from build123d import *

# Parameters (mm, degrees)
BOTTOM_PLATE_W                       = 140
BOTTOM_PLATE_H                       = 110
BOTTOM_PLATE_EXT_DEPTH               = 2
TOP_ROW_R                            = 8.25
TOP_ROW_R_2                          = 6.5
TOP_ROW_CUT_DEPTH                    = 179.056170912
SKETCH2_R                            = 6.5
SKETCH2_R_2                          = 3.55
BOTTOM_ROW_CUT_DEPTH                 = 10
SKETCH3_R                            = 6.5
CENTER_ROW_CUT_DEPTH                 = 10
PLATE_SCREWS_R                       = 1.65
PLATE_SCREWS_CUT_DEPTH               = 179.056170912
PLATE_SCREW_HEAD_R                   = 2.8
PLATE_SCREW_HEAD_CUT_DEPTH           = 2
PLATE_SCREW_HEAD_CUT_DRAFT           = -45
PLATE_SCREW_HEAD_CUT_PROFILE_2_DEPTH = 2
PLATE_SCREW_HEAD_CUT_PROFILE_2_DRAFT = -45
PLATE_SCREW_HEAD_CUT_PROFILE_3_DEPTH = 2
PLATE_SCREW_HEAD_CUT_PROFILE_3_DRAFT = -45
PLATE_SCREW_HEAD_CUT_PROFILE_4_DEPTH = 2
PLATE_SCREW_HEAD_CUT_PROFILE_4_DRAFT = -45
PLATE_SCREW_HEAD_CUT_PROFILE_5_DEPTH = 2
PLATE_SCREW_HEAD_CUT_PROFILE_5_DRAFT = -45
PLATE_SCREW_HEAD_CUT_PROFILE_6_DEPTH = 2
PLATE_SCREW_HEAD_CUT_PROFILE_6_DRAFT = -45
FILLET1_R                            = 2
FILLET2_R                            = 2
FILLET3_R                            = 2
FILLET4_R                            = 2


with BuildPart() as part:
    # Bottom Plate → Bottom Plate EXT (new body)
    with BuildSketch(Plane(origin=(0, 0, 0), x_dir=(1, 0, 0), z_dir=(0, 1, 0))):
        with Locations((-70, 55)):
            Rectangle(BOTTOM_PLATE_W, BOTTOM_PLATE_H)
    extrude(amount=BOTTOM_PLATE_EXT_DEPTH)

    # Top Row → Top Row Cut (cut, through all)
    with BuildSketch(Plane(origin=(0, 2, 0), x_dir=(1, 0, 0), z_dir=(0, 1, 0))):
        with Locations(Location((-123, 90, 0), (0, 0, 270))):
            Circle(TOP_ROW_R)
        with Locations(Location((-87.666666667, 90, 0), (0, 0, 270))):
            Circle(TOP_ROW_R_2)
        with Locations(Location((-52.333333333, 90, 0), (0, 0, 270))):
            Circle(TOP_ROW_R_2)
        with Locations(Location((-17, 90, 0), (0, 0, 270))):
            Circle(TOP_ROW_R_2)
    extrude(amount=-TOP_ROW_CUT_DEPTH, mode=Mode.SUBTRACT)

    # Sketch2 → Bottom Row Cut (cut)
    with BuildSketch(Plane(origin=(0, 2, 0), x_dir=(1, 0, 0), z_dir=(0, 1, 0))):
        with Locations(Location((-123, 20, 0), (0, 0, 270))):
            Circle(SKETCH2_R)
        with Locations(Location((-87.666666667, 20, 0), (0, 0, 270))):
            Circle(SKETCH2_R_2)
        with Locations(Location((-52.333333333, 20, 0), (0, 0, 270))):
            Circle(SKETCH2_R_2)
        with Locations(Location((-17, 20, 0), (0, 0, 270))):
            Circle(SKETCH2_R_2)
    extrude(amount=-BOTTOM_ROW_CUT_DEPTH, mode=Mode.SUBTRACT)

    # Sketch3 → Center Row Cut (cut)
    with BuildSketch(Plane(origin=(0, 2, 0), x_dir=(1, 0, 0), z_dir=(0, 1, 0))):
        with Locations(Location((-123, 55, 0), (0, 0, 270))):
            Circle(SKETCH3_R)
        with Locations(Location((-87.666666667, 55, 0), (0, 0, 270))):
            Circle(SKETCH3_R)
        with Locations(Location((-52.333333333, 55, 0), (0, 0, 270))):
            Circle(SKETCH3_R)
        with Locations(Location((-17, 55, 0), (0, 0, 270))):
            Circle(SKETCH3_R)
    extrude(amount=-CENTER_ROW_CUT_DEPTH, mode=Mode.SUBTRACT)

    # Plate Screws → Plate Screws Cut (cut, through all)
    with BuildSketch(Plane(origin=(0, 2, 0), x_dir=(1, 0, 0), z_dir=(0, 1, 0))):
        with Locations(Location((-135, 105, 0), (0, 0, 270))):
            Circle(PLATE_SCREWS_R)
        with Locations(Location((-5, 105, 0), (0, 0, 270))):
            Circle(PLATE_SCREWS_R)
        with Locations(Location((-5, 5, 0), (0, 0, 270))):
            Circle(PLATE_SCREWS_R)
        with Locations(Location((-135, 5, 0), (0, 0, 270))):
            Circle(PLATE_SCREWS_R)
        with Locations(Location((-70, 105, 0), (0, 0, 270))):
            Circle(PLATE_SCREWS_R)
        with Locations(Location((-70, 5, 0), (0, 0, 90))):
            Circle(PLATE_SCREWS_R)
    extrude(amount=-PLATE_SCREWS_CUT_DEPTH, mode=Mode.SUBTRACT)


with BuildPart() as plate_screw_head_cut_tool:
    # Plate Screw Head → Plate Screw Head Cut (with draft: the straight prism first)
    with BuildSketch(Plane(origin=(0, 2, 0), x_dir=(1, 0, 0), z_dir=(0, 1, 0))):
        with Locations((-135, 105)):
            Circle(PLATE_SCREW_HEAD_R)
    extrude(amount=-PLATE_SCREW_HEAD_CUT_DEPTH)
    # Plate Screw Head Cut: the draft: its side faces are tilted about the plane it starts from
    plate_screw_head_cut_sides = [plate_screw_head_cut_tool.faces().sort_by_distance(p)[0] for p in [
        (-137.8, 1, -105),
    ]]
    draft(plate_screw_head_cut_sides, Plane(origin=(0, 2, 0), x_dir=(1, 0, 0), z_dir=(0, 1, 0)), PLATE_SCREW_HEAD_CUT_DRAFT)


with BuildPart() as part_1:
    add(part.part)

    # Plate Screw Head Cut: cut by plate_screw_head_cut_tool
    add(plate_screw_head_cut_tool.part, mode=Mode.SUBTRACT)


with BuildPart() as plate_screw_head_cut_profile_2_tool:
    # Plate Screw Head → Plate Screw Head Cut profile 2 (with draft: the straight prism first)
    with BuildSketch(Plane(origin=(0, 2, 0), x_dir=(1, 0, 0), z_dir=(0, 1, 0))):
        with Locations((-5, 105)):
            Circle(PLATE_SCREW_HEAD_R)
    extrude(amount=-PLATE_SCREW_HEAD_CUT_PROFILE_2_DEPTH)
    # Plate Screw Head Cut profile 2: the draft: its side faces are tilted about the plane it starts from
    plate_screw_head_cut_profile_2_sides = [plate_screw_head_cut_profile_2_tool.faces().sort_by_distance(p)[0] for p in [
        (-7.8, 1, -105),
    ]]
    draft(plate_screw_head_cut_profile_2_sides, Plane(origin=(0, 2, 0), x_dir=(1, 0, 0), z_dir=(0, 1, 0)), PLATE_SCREW_HEAD_CUT_PROFILE_2_DRAFT)


with BuildPart() as part_2:
    add(part_1.part)

    # Plate Screw Head Cut profile 2: cut by plate_screw_head_cut_profile_2_tool
    add(plate_screw_head_cut_profile_2_tool.part, mode=Mode.SUBTRACT)


with BuildPart() as plate_screw_head_cut_profile_3_tool:
    # Plate Screw Head → Plate Screw Head Cut profile 3 (with draft: the straight prism first)
    with BuildSketch(Plane(origin=(0, 2, 0), x_dir=(1, 0, 0), z_dir=(0, 1, 0))):
        with Locations((-5, 5)):
            Circle(PLATE_SCREW_HEAD_R)
    extrude(amount=-PLATE_SCREW_HEAD_CUT_PROFILE_3_DEPTH)
    # Plate Screw Head Cut profile 3: the draft: its side faces are tilted about the plane it starts from
    plate_screw_head_cut_profile_3_sides = [plate_screw_head_cut_profile_3_tool.faces().sort_by_distance(p)[0] for p in [
        (-7.8, 1, -5),
    ]]
    draft(plate_screw_head_cut_profile_3_sides, Plane(origin=(0, 2, 0), x_dir=(1, 0, 0), z_dir=(0, 1, 0)), PLATE_SCREW_HEAD_CUT_PROFILE_3_DRAFT)


with BuildPart() as part_3:
    add(part_2.part)

    # Plate Screw Head Cut profile 3: cut by plate_screw_head_cut_profile_3_tool
    add(plate_screw_head_cut_profile_3_tool.part, mode=Mode.SUBTRACT)


with BuildPart() as plate_screw_head_cut_profile_4_tool:
    # Plate Screw Head → Plate Screw Head Cut profile 4 (with draft: the straight prism first)
    with BuildSketch(Plane(origin=(0, 2, 0), x_dir=(1, 0, 0), z_dir=(0, 1, 0))):
        with Locations((-135, 5)):
            Circle(PLATE_SCREW_HEAD_R)
    extrude(amount=-PLATE_SCREW_HEAD_CUT_PROFILE_4_DEPTH)
    # Plate Screw Head Cut profile 4: the draft: its side faces are tilted about the plane it starts from
    plate_screw_head_cut_profile_4_sides = [plate_screw_head_cut_profile_4_tool.faces().sort_by_distance(p)[0] for p in [
        (-137.8, 1, -5),
    ]]
    draft(plate_screw_head_cut_profile_4_sides, Plane(origin=(0, 2, 0), x_dir=(1, 0, 0), z_dir=(0, 1, 0)), PLATE_SCREW_HEAD_CUT_PROFILE_4_DRAFT)


with BuildPart() as part_4:
    add(part_3.part)

    # Plate Screw Head Cut profile 4: cut by plate_screw_head_cut_profile_4_tool
    add(plate_screw_head_cut_profile_4_tool.part, mode=Mode.SUBTRACT)


with BuildPart() as plate_screw_head_cut_profile_5_tool:
    # Plate Screw Head → Plate Screw Head Cut profile 5 (with draft: the straight prism first)
    with BuildSketch(Plane(origin=(0, 2, 0), x_dir=(1, 0, 0), z_dir=(0, 1, 0))):
        with Locations((-70, 105)):
            Circle(PLATE_SCREW_HEAD_R)
    extrude(amount=-PLATE_SCREW_HEAD_CUT_PROFILE_5_DEPTH)
    # Plate Screw Head Cut profile 5: the draft: its side faces are tilted about the plane it starts from
    plate_screw_head_cut_profile_5_sides = [plate_screw_head_cut_profile_5_tool.faces().sort_by_distance(p)[0] for p in [
        (-72.8, 1, -105),
    ]]
    draft(plate_screw_head_cut_profile_5_sides, Plane(origin=(0, 2, 0), x_dir=(1, 0, 0), z_dir=(0, 1, 0)), PLATE_SCREW_HEAD_CUT_PROFILE_5_DRAFT)


with BuildPart() as part_5:
    add(part_4.part)

    # Plate Screw Head Cut profile 5: cut by plate_screw_head_cut_profile_5_tool
    add(plate_screw_head_cut_profile_5_tool.part, mode=Mode.SUBTRACT)


with BuildPart() as plate_screw_head_cut_profile_6_tool:
    # Plate Screw Head → Plate Screw Head Cut profile 6 (with draft: the straight prism first)
    with BuildSketch(Plane(origin=(0, 2, 0), x_dir=(1, 0, 0), z_dir=(0, 1, 0))):
        with Locations((-70, 5)):
            Circle(PLATE_SCREW_HEAD_R)
    extrude(amount=-PLATE_SCREW_HEAD_CUT_PROFILE_6_DEPTH)
    # Plate Screw Head Cut profile 6: the draft: its side faces are tilted about the plane it starts from
    plate_screw_head_cut_profile_6_sides = [plate_screw_head_cut_profile_6_tool.faces().sort_by_distance(p)[0] for p in [
        (-72.8, 1, -5),
    ]]
    draft(plate_screw_head_cut_profile_6_sides, Plane(origin=(0, 2, 0), x_dir=(1, 0, 0), z_dir=(0, 1, 0)), PLATE_SCREW_HEAD_CUT_PROFILE_6_DRAFT)


with BuildPart() as part_6:
    add(part_5.part)

    # Plate Screw Head Cut profile 6: cut by plate_screw_head_cut_profile_6_tool
    add(plate_screw_head_cut_profile_6_tool.part, mode=Mode.SUBTRACT)

    # Fillet1
    fillet1_edges = [part_6.edges().sort_by_distance(p)[0] for p in [
        (-140, 1, -110),
    ]]
    fillet(fillet1_edges, radius=FILLET1_R)

    # Fillet2
    fillet2_edges = [part_6.edges().sort_by_distance(p)[0] for p in [
        (0, 1, -110),
    ]]
    fillet(fillet2_edges, radius=FILLET2_R)

    # Fillet3
    fillet3_edges = [part_6.edges().sort_by_distance(p)[0] for p in [
        (0, 1, 0),
    ]]
    fillet(fillet3_edges, radius=FILLET3_R)

    # Fillet4
    fillet4_edges = [part_6.edges().sort_by_distance(p)[0] for p in [
        (-140, 1, 0),
    ]]
    fillet(fillet4_edges, radius=FILLET4_R)


solid = part_6.part
The listing builds one solid part. Answer for the finished solid, in the listing's coordinates (mm). Round coordinates to 2 decimals unless told otherwise and drop trailing zeros. Order: outer loops, then holes, each group sorted by start corner. A loop starts at its lowest first (then second) coordinate and runs counter-clockwise, first axis right, second up. Notation, with made-up numbers: (-13, -31.75) -> (28, -31.75) arc R31 ccw to (28, 5.25) -> close; hole circle Ø3 at (-0.75, 41). An arc over 180 degrees is marked (long way). One line per item, written item: value.
Item 1: Straight lines are drawn through the part: L1, parallel to Z at x = -5, y = 0.5; L2, parallel to X at y = 0.6, z = -105; L3, parallel to X at y = 1.45, z = -20. For each, find the intervals that lie inside material, in ascending order.
Taken from the geometry:
L1: z = -110 to -106.65, -103.35 to -6.65, -3.35 to 0
L2: x = -140 to -136.65, -133.35 to -71.65, -68.35 to -6.65, -3.35 to 0
L3: x = -140 to -129.5, -116.5 to -91.22, -84.12 to -55.88, -48.78 to -20.55, -13.45 to 0
Item 2: Find section D-D, the plane y = 1.35. State how many separate pieces and enclosed holes the cut face has, then the cut area to 3 significant figures.
Taken from the geometry:
separate pieces: 1
enclosed holes: 18
area: 13,900 mm2
Item 3: Find section B-B, the plane x = -123. Give the vertices of the cut face in (y, z), then the cut area to 3 significant figures.
Taken from the geometry:
outline: (0, -110) -> (2, -110) -> (2, -98.25) -> (0, -98.25) -> close; (0, -81.75) -> (2, -81.75) -> (2, -61.5) -> (0, -61.5) -> close; (0, -48.5) -> (2, -48.5) -> (2, -26.5) -> (0, -26.5) -> close; (0, -13.5) -> (2, -13.5) -> (2, 0) -> (0, 0) -> close
area: 135 mm2
Item 4: For a pull along Z with two mould halves and no side action, classify faces 1 (the flat face through (-71, 2, -56)), 2 (the cylindrical face through (-91.132, 1.014, -20.77)) as released by +Z, released by -Z, zero draft, split by the parting line, or undercut.
Taken from the geometry:
face 1: zero draft
face 2: undercut
Item 5: Given P1, Ø5.5, axis at x = -70, z = -105, coming from the +Y side; P2, Ø8, axis at x = -17, z = -55, coming from the +Y side, each flat-ended and moving along its own axis, determine where each tip first touches the part or whether it passes through.
Taken from the geometry:
P1: stops at y = 1.95
P2: passes through
Item 6: Find section C-C, the plane z = -105. Give the vertices of the cut face in (x, y).
Taken from the geometry:
outline: (-140, 0) -> (-136.65, 0) -> (-136.65, 0.85) -> (-137.8, 2) -> (-140, 2) -> close; (-133.35, 0) -> (-71.65, 0) -> (-71.65, 0.85) -> (-72.8, 2) -> (-132.2, 2) -> (-133.35, 0.85) -> close; (-68.35, 0) -> (-6.65, 0) -> (-6.65, 0.85) -> (-7.8, 2) -> (-67.2, 2) -> (-68.35, 0.85) -> close; (-3.35, 0) -> (0, 0) -> (0, 2) -> (-2.2, 2) -> (-3.35, 0.85) -> close
Item 7: Find section A-A, the plane z = -20. Give the vertices of the cut face in (x, y), then the cut area to 3 significant figures.
Taken from the geometry:
outline: (-140, 0) -> (-129.5, 0) -> (-129.5, 2) -> (-140, 2) -> close; (-116.5, 0) -> (-91.22, 0) -> (-91.22, 2) -> (-116.5, 2) -> close; (-84.12, 0) -> (-55.88, 0) -> (-55.88, 2) -> (-84.12, 2) -> close; (-48.78, 0) -> (-20.55, 0) -> (-20.55, 2) -> (-48.78, 2) -> close; (-13.45, 0) -> (0, 0) -> (0, 2) -> (-13.45, 2) -> close
area: 211 mm2
